Input: part model. Units: mm. Frame: model coordinates. A direction names the side the tool comes from. Coordinates: 2 decimals unless noted, no trailing zeros. Write each loop counter-clockwise with the first axis right and the second up, starting at its lowest first coordinate (ties: lowest second). Pieces come first, ordered by that corner, then holes. Notation, with made-up numbers: M 42,10 L 88,10 A20 ccw 88,49 Z; hole C -22.75,29.5 d5. An arc over 180 degrees is marked long. Use one line per item in the form item = value.
from build123d import *

# Parameters (mm, degrees)
F0_W     = 40
F0_H     = 40
F0_R     = 1.75
F1_DEPTH = 10
F2_R     = 3.1
F3_DEPTH = 3
F4_W     = 5.6
F4_H     = 8
F5_DEPTH = 2.5
F6_SIZE  = 0.5
F7_SIZE  = 0.5


with BuildPart() as f1:
    # F0 (on Top) → F1 (new body)
    with BuildSketch(Plane.XY):
        Rectangle(F0_W, F0_H)
        with Locations((-10, -10)):
            Circle(F0_R, mode=Mode.SUBTRACT)
        with Locations((10, -10)):
            Circle(F0_R, mode=Mode.SUBTRACT)
        with Locations((-10, 10)):
            Circle(F0_R, mode=Mode.SUBTRACT)
        with Locations((10, 10)):
            Circle(F0_R, mode=Mode.SUBTRACT)
    extrude(amount=F1_DEPTH)

    # F2 (on face) → F3 (cut)
    with BuildSketch(Plane(origin=(0, 0, 0), x_dir=(1, 0, 0), z_dir=(0, 0, -1))):
        with Locations((10, 10)):
            Circle(F2_R)
        with Locations((10, -10)):
            Circle(F2_R)
        with Locations((-10, -10)):
            Circle(F2_R)
        with Locations((-10, 10)):
            Circle(F2_R)
    extrude(amount=-F3_DEPTH, mode=Mode.SUBTRACT)

    # F4 (on face) → F5 (cut)
    with BuildSketch(Plane.XY.offset(10)):
        with Locations((-10, 10)):
            Rectangle(F4_W, F4_H)
        with Locations((10, 10)):
            Rectangle(F4_W, F4_H)
        with Locations((10, -10)):
            Rectangle(F4_W, F4_H)
        with Locations((-10, -10)):
            Rectangle(F4_W, F4_H)
    extrude(amount=-F5_DEPTH, mode=Mode.SUBTRACT)

    # F6
    f6_edges = [f1.edges().sort_by_distance(p)[0] for p in [
        (-20, 0, 10),
        (0, 20, 10),
        (20, 0, 10),
        (0, -20, 10),
        (12.8, -10, 10),
        (10, -14, 10),
        (7.2, -10, 10),
        (10, -6, 10),
        (-7.2, -10, 10),
        (-12.8, -10, 10),
        (-10, -6, 10),
        (-10, -14, 10),
        (-10, 14, 10),
        (-12.8, 10, 10),
        (-10, 6, 10),
        (-7.2, 10, 10),
        (12.8, 10, 10),
        (10, 14, 10),
        (7.2, 10, 10),
        (10, 6, 10),
    ]]
    chamfer(f6_edges, length=F6_SIZE)

    # F7
    f7_edges = [f1.edges().sort_by_distance(p)[0] for p in [
        (6.9, -10, 0),
        (-13.1, -10, 0),
        (6.9, 10, 0),
        (-13.1, 10, 0),
        (8.25, -10, 3),
        (-11.75, -10, 3),
        (8.25, 10, 3),
        (-11.75, 10, 3),
        (-20, 0, 0),
        (0, 20, 0),
        (0, -20, 0),
        (20, 0, 0),
        (8.25, 10, 7.5),
        (8.25, -10, 7.5),
        (-11.75, 10, 7.5),
        (-11.75, -10, 7.5),
    ]]
    chamfer(f7_edges, length=F7_SIZE)


solid = f1.part
(1) Line query: probe 1 along X at (y, z) = (10, 1.8); probe 2 along X at (y, z) = (-10, 5.55). Output: solid intervals per line, ascending.
Computed:
probe_1 = -20 to -13.1, -6.9 to 6.9, 13.1 to 20
probe_2 = -20 to -11.75, -8.25 to 8.25, 11.75 to 20
(2) Section query C-C on z = 1.75. Return the cut outline in (x, y).
Computed:
outline = M -20,-20 L 20,-20 L 20,20 L -20,20 Z; hole C -10,-10 d6.2; hole C -10,10 d6.2; hole C 10,-10 d6.2; hole C 10,10 d6.2
(3) Section query B-B on x = 10. State how many separate pieces and enclosed holes the cut face has, plus the area to 3 significant figures.
Computed:
separate_pieces = 3
enclosed_holes = 0
area = 289 mm^2
(4) First-contact query: pin 1 Ø1.9 at (x, y) = (-10.5, 11) entering from -Z; pin 2 Ø12 at (x, y) = (8.5, -2.5) entering from -Z; pin 3 Ø5 at (x, y) = (10.5, -10.5) entering from -Z. Flat tips, straight axial feed; report the tip coordinate or a pass-through.
Computed:
pin_1 = 3.18
pin_2 = 0
pin_3 = 0.39
(5) Section query A-A on z = 6.5. Return the cut outline in (x, y).
Computed:
outline = M -20,-20 L 20,-20 L 20,20 L -20,20 Z; hole C -10,-10 d3.5; hole C -10,10 d3.5; hole C 10,-10 d3.5; hole C 10,10 d3.5
(6) Pull-direction query (Y, two-part tool) for faces 4 (the flat face through (20, 0, 5)), 5 (the flat face through (12, -12, 3)); classes: pulls with the +Y half, pulls with the -Y half, needs draft (parallel to the pull), parting line crosses it, or undercut.
Computed:
face_4 = needs draft
face_5 = undercut
(7) Set-up query: faces 1 (the flat face through (0, 0, 10)), 2 (the cylindrical face through (6.9, 9.9, 1.7)), 3 (the flat face through (10, -6, 9)). Return all of +Z, -Z, +X, -X, +Y, -Y with unobstructed straight access to the full face (end or side cutting, diameter ignored); none if empty.
Computed:
face_1 = +Z, +X, -X, +Y, -Y
face_2 = -Z
face_3 = +Z
